Part print with two shaded views. Sizes in mm from the minimum x, y, z corner. A direction names the side the tool comes from. Round coordinates to 2 decimals unless told otherwise and drop trailing zeros. Loops run counter-clockwise (first coordinate to the right, second up) from the corner with the lowest first, then second, coordinate; pieces in that order, holes last.
(1) Cut at B-B on z = 50.5. List the corners of the cut face in (x, y).
(2) Mould opens along X. For the marked faces 4, 5 and 6 say: +X half, -X half, draft (parallel to the pull), parting line (faces both ways), or undercut.
(3) Cut at D-D on x = 112. List the corners of the cut face in (y, z).
(4) Tool access for the marked faces 1, 2 and 3: list every direction of +Z, -Z, +X, -X, +Y, -Y with a clear straight run to the whole face (end or side of a thin tool).
(5) Cut at A-A on y = 22. List the corners of the cut face in (x, z).
(6) Flat gauge pins, fed straight in: pin 1 (4 mm diameter, centred on x = 56, y = 23.5, fed in from +Z); pin 2 (2.5 mm diameter, centred on x = 111.5, y = 8, fed in from +Z); pin 3 (8 mm diameter, centred on y = 27, z = 39, fed in from -X). Where does each tip first touch, or does it go through?
(7) Probe probe 1 along X at (y, z) = (34.5, 25.5); probe 2 along X at (y, z) = (13.5, 10.5); probe 3 along Y at (x, z) = (68, 50.5). List the from-to ranges inside material, lowest first.
(8) Cut at C-C on x = 7. List the corners of the cut face in (y, z).
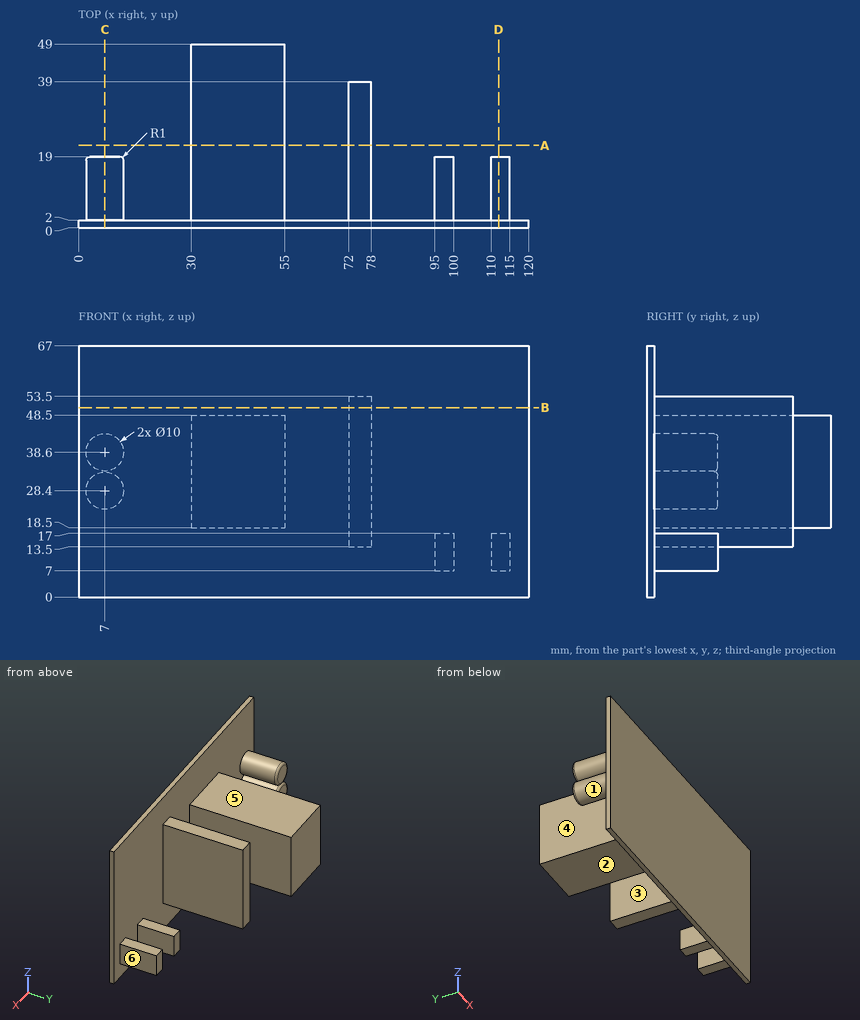
Final values:
1. outline: (0, 0) - (120, 0) - (120, 2) - (78, 2) - (78, 39) - (72, 39) - (72, 2) - (0, 2) - close
2. face 4: undercut
2. face 5: draft
2. face 6: +X half
3. outline: (0, 0) - (2, 0) - (2, 7) - (19, 7) - (19, 17) - (2, 17) - (2, 67) - (0, 67) - close
4. face 1: +Y
4. face 2: -Z, -X, +Y
4. face 3: +Z, -Z, +Y
5. outline: (30, 18.5) - (55, 18.5) - (55, 48.5) - (30, 48.5) - close; (72, 13.5) - (78, 13.5) - (78, 53.5) - (72, 53.5) - close
6. pin 1: stops at z = 48.5
6. pin 2: stops at z = 17
6. pin 3: stops at x = 30
7. probe 1: x = 30 to 55, 72 to 78
7. probe 2: x = 95 to 100, 110 to 115
7. probe 3: y = 0 to 2
8. outline: (0, 0) - (2, 0) - (2, 23.4) - (18, 23.4) arc R1 ccw to (19, 24.4) - (19, 32.4) arc R1 ccw to (18, 33.4) - (2, 33.4) - (2, 33.6) - (18, 33.6) arc R1 ccw to (19, 34.6) - (19, 42.6) arc R1 ccw to (18, 43.6) - (2, 43.6) - (2, 67) - (0, 67) - close
